Answer from the drawing. Dimensions are ordinates in mm from the lowest x, y and z of the part. A direction names the side the tool comes from. Coordinates: 2 decimals unless noted, no trailing zeros. Order: outer loops, then holes, each group sorted by start corner. A loop starts at its lowest first (then second) coordinate and runs counter-clockwise, first axis right, second up. Notation, with made-up numbers: (-5.75, -12.75) -> (43.25, -12.75) arc R14 ccw to (43.25, 5.25) -> close; hole circle Ø9 at (32.25, -16). An arc over 180 degrees is marked (long way). Answer in a Markdown table with one row per item.
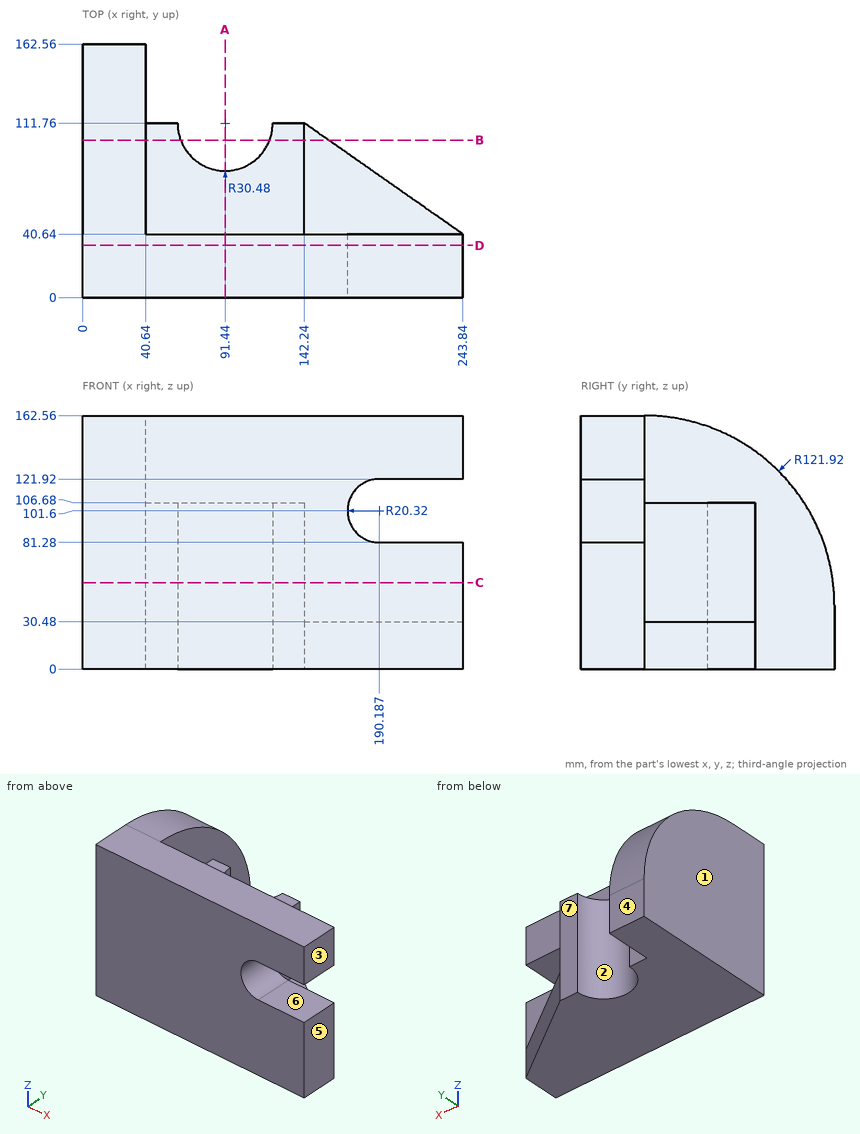
(1) For a pull along X with two mould halves and no side action, classify the marked faces 1, 2, 3 and 4 as released by +X, released by -X, zero draft, split by the parting line, or undercut.
Check values:
| item | result |
|---|---|
| face 1 | released by -X |
| face 2 | undercut |
| face 3 | released by +X |
| face 4 | zero draft |
(2) Find the intervals of material crossed by line 1 along X through (y, z) = (122, 52); line 2 along X through (y, z) = (44.5, 79); line 3 along Z through (x, y) = (97, 48), in increasing order. Write a range as from..to.
Check values:
| item | result |
|---|---|
| line 1 | 0..40.64 |
| line 2 | 0..142.24 |
| line 3 | 0..106.68 |
(3) Which of the six approach directions +Z, -Z, +X, -X, +Y, -Y give full straight-line access (tool end or side, diameter ignored) to the marked faces 5, 6 and 7?
Check values:
| item | result |
|---|---|
| face 5 | +Z, -Z, +X, +Y, -Y |
| face 6 | +X, +Y, -Y |
| face 7 | +Z, -Z, +X, +Y |
(4) A cutting plane is placed at A-A, the plane x = 91.44. Determine the outline of the cut face in (y, z).
Check values:
| item | result |
|---|---|
| outline | (0, 0) -> (81.28, 0) -> (81.28, 106.68) -> (40.64, 106.68) -> (40.64, 162.56) -> (0, 162.56) -> close |
(5) A cutting plane is placed at B-B, the plane y = 101. Determine the outline of the cut face in (x, z).
Check values:
| item | result |
|---|---|
| outline | (0, 0) -> (62.92, 0) -> (62.92, 106.68) -> (40.64, 106.68) -> (40.64, 146.57) -> (0, 146.57) -> close; (119.96, 0) -> (157.61, 0) -> (157.61, 30.48) -> (142.24, 30.48) -> (142.24, 106.68) -> (119.96, 106.68) -> close |
(6) A cutting plane is placed at D-D, the plane y = 33.5. Determine the outline of the cut face in (x, z), then the cut area to 3 significant figures.
Check values:
| item | result |
|---|---|
| outline | (0, 0) -> (243.84, 0) -> (243.84, 81.28) -> (190.19, 81.28) arc R20.32 cw to (190.19, 121.92) -> (243.84, 121.92) -> (243.84, 162.56) -> (0, 162.56) -> close |
| area | 36,800 mm² |
(7) Flat-ended cylindrical pins translate along their axes: pin 1 (1.5 mm diameter, centred on x = 39, z = 122.5, fed in from +Y) (1 decimal); pin 2 (2 mm diameter, centred on x = 153, z = 41, fed in from +Y); pin 3 (10 mm diameter, centred on x = 133.5, z = 29.5, fed in from +Y); pin 4 (10 mm diameter, centred on x = 211, z = 87, fed in from +Y). Find the tip coordinate at first contact, or state that the pin passes through.
Check values:
| item | result |
|---|---|
| pin 1 | y = 131.7 |
| pin 2 | y = 40.64 |
| pin 3 | y = 111.76 |
| pin 4 | through |
(8) A cutting plane is placed at C-C, the plane z = 55.5. Determine the outline of the cut face in (x, y).
Check values:
| item | result |
|---|---|
| outline | (0, 0) -> (243.84, 0) -> (243.84, 40.64) -> (142.24, 40.64) -> (142.24, 111.76) -> (121.92, 111.76) arc R30.48 cw to (60.96, 111.76) -> (40.64, 111.76) -> (40.64, 161.65) -> (0, 161.65) -> close |
